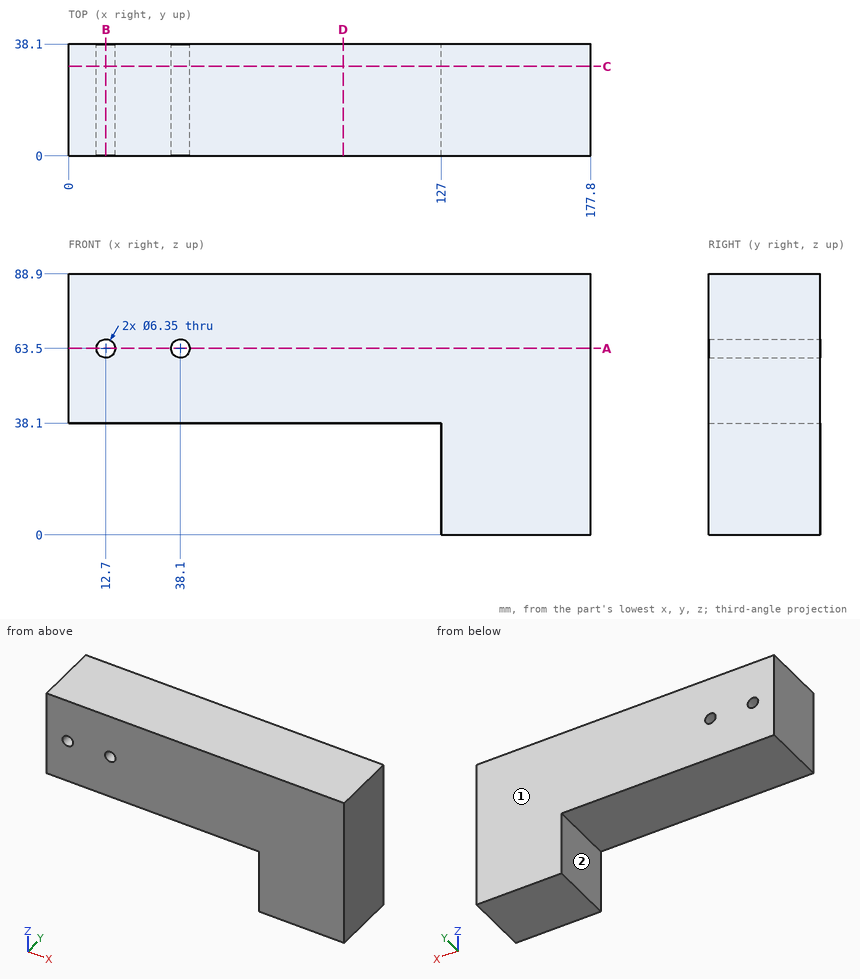
Could you check a few things on this drawing? It's one solid part, dimensions in mm from its lowest x, y, z. A direction names the side the tool comes from. Round coordinates to 2 decimals unless told otherwise and drop trailing zeros. Order: outer loops, then holes, each group sorted by start corner. A loop starts at its lowest first (then second) coordinate and runs counter-clockwise, first axis right, second up. Notation, with made-up numbers: M -6,36.5 L 16,36.5 A15 ccw 16,59.5 Z; hole C -4.75,75.5 d3. An arc over 180 degrees is marked long. One line per item, written item: value.
(1) Which directions (+Z, -Z, +X, -X, +Y, -Y) give clear straight access to the entire face, cutting with the end or side of a thin tool? Please do the marked faces 1 and 2.
Ans:
face 1: +Z, -Z, +X, -X, +Y
face 2: -Z, -X, +Y, -Y
(2) I'm going to push flat-ended pins straight in: P1, Ø1, axis at y = 18.5, z = 37, coming from the -X side; P2, Ø4, axis at y = 25, z = 36.5, coming from the -X side; P3, Ø2, axis at x = 114, y = 5.5, coming from the -Z side. Where does each tip first touch, or does it pass through?
Ans:
P1: stops at x = 127
P2: stops at x = 0
P3: stops at z = 38.1
(3) Imagine slicing it at D-D (x = 93.5). Write out the boundary of the cut face in (y, z), and give its area (3 significant figures).
Ans:
outline: M 0,38.1 L 38.1,38.1 L 38.1,88.9 L 0,88.9 Z
area: 1,940 mm^2
(4) Imagine slicing it at A-A (z = 63.5). Write out the boundary of the cut face in (x, y) (3 decimals).
Ans:
outline: M 0,0 L 9.525,0 L 9.525,38.1 L 0,38.1 Z; M 15.875,0 L 34.925,0 L 34.925,38.1 L 15.875,38.1 Z; M 41.275,0 L 177.8,0 L 177.8,38.1 L 41.275,38.1 Z
(5) I need wall thicknesses on line 1 along Z through (x, y) = (38.1, 23) (3 decimals); line 2 along X through (y, z) = (3, 30.5); line 3 along Z through (x, y) = (43.5, 8.5). Which ranges of each line are inside material? Lowest first, please. Write a range as from..to.
Ans:
line 1: z = 38.1..60.325, 66.675..88.9
line 2: x = 127..177.8
line 3: z = 38.1..88.9
(6) Imagine slicing it at B-B (x = 12.7). Write out the boundary of the cut face in (y, z) (3 decimals), and give its area (3 significant figures).
Ans:
outline: M 0,38.1 L 38.1,38.1 L 38.1,60.325 L 0,60.325 Z; M 0,66.675 L 38.1,66.675 L 38.1,88.9 L 0,88.9 Z
area: 1,690 mm^2
(7) Imagine slicing it at C-C (y = 30.5). Write out the boundary of the cut face in (x, z) (3 decimals), and give its area (3 significant figures).
Ans:
outline: M 0,38.1 L 127,38.1 L 127,0 L 177.8,0 L 177.8,88.9 L 0,88.9 Z; hole C 12.7,63.5 d6.35; hole C 38.1,63.5 d6.35
area: 10,900 mm^2
